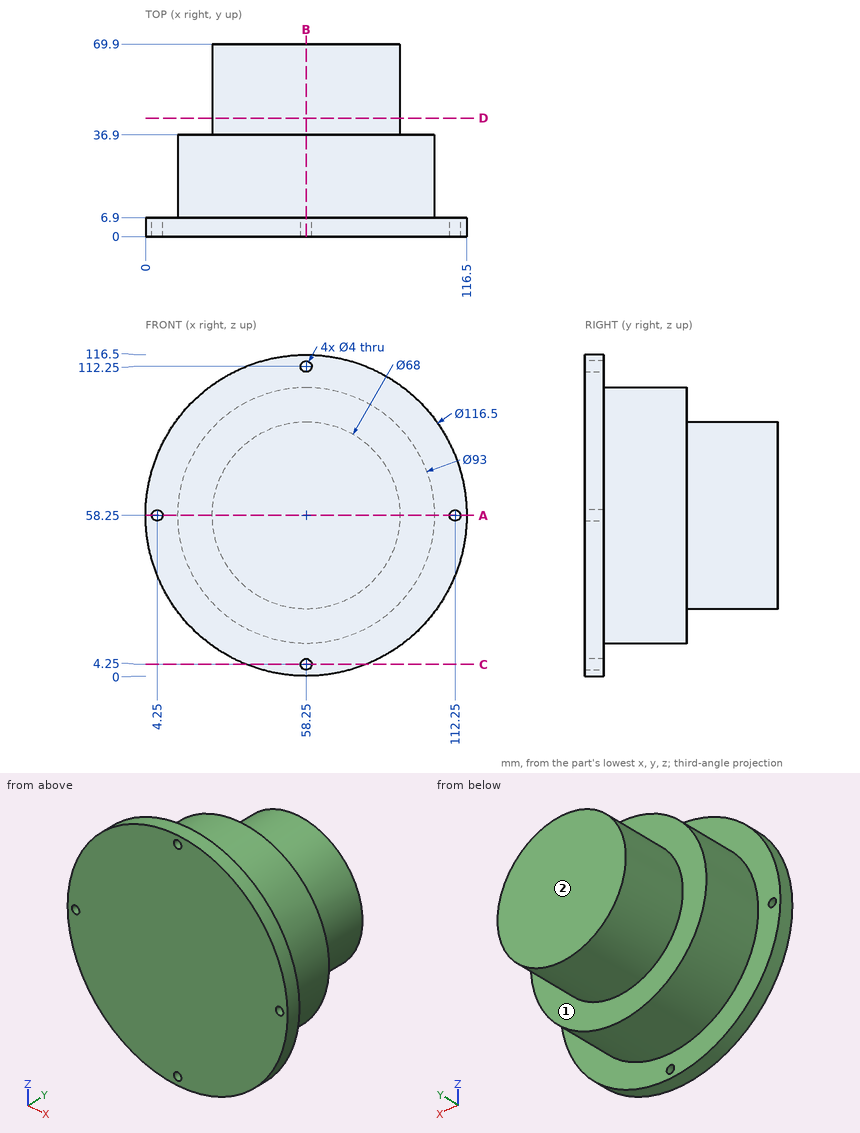
For this review, use the dimensioned drawing (mm, ordinates from the lowest corner) and the shaded views. A direction names the side the tool comes from. Give positions to 0.01 mm unless a question says otherwise; leave off trailing zeros. Loops run counter-clockwise (first coordinate to the right, second up) from the corner with the lowest first, then second, coordinate; pieces in that order, holes last.
Item 1: Insertion check: pin 1 (1.5 mm diameter, centred on y = 31, z = 58, fed in from -X); pin 2 (4.5 mm diameter, centred on x = 58.25, z = 112.25, fed in from +Y); pin 3 (6 mm diameter, centred on y = 31, z = 98.5, fed in from +X). Each pin has a flat end and moves straight along its axis. Give the tip position at first contact, or say it passes through.
Item 2: Take a section at B-B, the plane x = 58.25. State the section outline as (y, z) points, and give its area (3 significant figures).
Item 3: For line 1 along X through (y, z) = (5.25, 58.25); line 2 along Z through (x, y) = (58, 4); line 3 along Z through (x, y) = (112.25, 5), list the stretches that pass through material, from the lowest coordinate up.
Item 4: Take a section at D-D, the plane y = 43. State the section outline as (x, z) points, and give its area (3 significant figures).
Item 5: Tool access review of the marked faces 1 and 2: name each direction out of +Z, -Z, +X, -X, +Y, -Y from which nothing blocks a thin tool from reaching the whole face with its end or side.
Item 6: Take a section at A-A, the plane z = 58.25. State the section outline as (x, y) points.
Item 7: Take a section at C-C, the plane z = 4.25. State the section outline as (x, y) points, and give its area (3 significant figures).
Calculated:
1. pin 1: stops at x = 11.75
1. pin 2: stops at y = 6.9
1. pin 3: stops at x = 86.08
2. outline: (0, 0) - (6.9, 0) - (6.9, 2.25) - (0, 2.25) - close; (0, 6.25) - (6.9, 6.25) - (6.9, 11.75) - (36.9, 11.75) - (36.9, 24.25) - (69.9, 24.25) - (69.9, 92.25) - (36.9, 92.25) - (36.9, 104.75) - (6.9, 104.75) - (6.9, 110.25) - (0, 110.25) - close; (0, 114.25) - (6.9, 114.25) - (6.9, 116.5) - (0, 116.5) - close
2. area: 5,780 mm2
3. line 1: x = 0 to 2.25, 6.25 to 110.25, 114.25 to 116.5
3. line 2: z = 0 to 2.27, 6.23 to 110.27, 114.23 to 116.5
3. line 3: z = 36.41 to 56.25, 60.25 to 80.09
4. outline: circle Ø68 at (58.25, 58.25)
4. area: 3,630 mm2
5. face 1: +Y
5. face 2: +Z, -Z, +X, -X, +Y
6. outline: (0, 0) - (2.25, 0) - (2.25, 6.9) - (0, 6.9) - close; (6.25, 0) - (110.25, 0) - (110.25, 6.9) - (104.75, 6.9) - (104.75, 36.9) - (92.25, 36.9) - (92.25, 69.9) - (24.25, 69.9) - (24.25, 36.9) - (11.75, 36.9) - (11.75, 6.9) - (6.25, 6.9) - close; (114.25, 0) - (116.5, 0) - (116.5, 6.9) - (114.25, 6.9) - close
7. outline: (36.41, 0) - (56.25, 0) - (56.25, 6.9) - (36.41, 6.9) - close; (60.25, 0) - (80.09, 0) - (80.09, 6.9) - (60.25, 6.9) - close
7. area: 274 mm2
